Autodesk Fusion 360 part; units mm, degrees
sketch "Sketch1" plane through (0, 0, 0) normal (0, 1, 0) x (1, 0, 0)
  line L0 (0, 0) -> (70, 0)
  line L1 (70, 0) -> (70, -50)
  line L2 (70, -50) -> (0, -50)
  line L3 (0, -50) -> (0, 0)
  circle A0 centre (0, -50) radius 2
  circle A1 centre (0, 0) radius 2
  circle A2 centre (70, 0) radius 2
  circle A3 centre (70, -50) radius 2
  line L4 (0, 4) -> (70, 4)
  line L5 (74, 0) -> (74, -50)
  line L6 (70, -54) -> (0, -54)
  line L7 (-4, -50) -> (-4, 0)
  arc A4 (-4, -50) -> (0, -54) centre (0, -50) ccw
  arc A5 (0, 4) -> (-4, 0) centre (0, 0) ccw
  arc A6 (70, -54) -> (74, -50) centre (70, -50) ccw
  arc A7 (74, 0) -> (70, 4) centre (70, 0) ccw
  dimension "d1" = 70
  dimension "d2" = 50
  dimension "d3" = 4
  dimension "d4" = 4
  dimension "d5" = 4
  dimension "d6" = 4
  dimension "d8" = 4
  dimension "d9" = 4
  dimension "d10" = 4
  dimension "d11" = 4
extrude "Extrude1" add sketch "Sketch1" along normal blind 1 contours L0 L1 L2 L3 A0 A1 A2 A3 | L4 L5 L6 L7 A4 A5 A6 A7
sketch "Sketch2" plane through (0, 0, 0) normal (0, -1, 0) x (1, 0, 0)
  circle A0 centre (0, 0) radius 2
  circle A1 centre (0, 50) radius 2
  circle A2 centre (70, 0) radius 2
  circle A3 centre (70, 50) radius 2
  arc A4 (74, 50) -> (70, 54) centre (70, 50) ccw
  line L0 (70, 54) -> (0, 54)
  arc A5 (0, 54) -> (-4, 50) centre (0, 50) ccw
  line L1 (-4, 50) -> (-4, 0)
  arc A6 (-4, 0) -> (0, -4) centre (0, 0) ccw
  line L2 (0, -4) -> (70, -4)
  arc A7 (70, -4) -> (74, 0) centre (70, 0) ccw
  line L3 (74, 0) -> (74, 50)
  line L4 (10, 54) -> (10, -4)
  line L5 (56.228, 54) -> (56.228, -4)
  circle A8 centre (10, 32.046) radius 1.15
  circle A9 centre (56.228, 38.142) radius 1.15
  circle A10 centre (56.228, 25.188) radius 1.15
  line L6 (10, 45) -> (56.228, 45)
  line L7 (56.228, 45) -> (56.228, 5)
  line L8 (56.228, 5) -> (10, 5)
  line L9 (10, 5) -> (10, 45)
  line L10 (10, 25) -> (-4, 25)
  circle A11 centre (10, 32.046) radius 3.15
  circle A12 centre (56.228, 38.142) radius 3.15
  circle A13 centre (56.228, 25.188) radius 3.15
  line L11 (56.228, 38.142) -> (56.228, 25.188)
  circle A14 centre (53.728, 31.665) radius 1.5
  circle A15 centre (58.728, 31.665) radius 1.5
  line L12 (0, 50) -> (70, 50)
  line L13 (32.5, 51.5) -> (37.5, 51.5)
  line L14 (37.5, 51.5) -> (37.5, 48.5)
  line L15 (37.5, 48.5) -> (32.5, 48.5)
  line L16 (32.5, 48.5) -> (32.5, 51.5)
  line L17 (32.5, 51.5) -> (37.5, 48.5)
  line L18 (32.5, 48.5) -> (37.5, 51.5)
  line L19 (53.728, 31.665) -> (58.728, 31.665)
  point P0 (35, 50)
  point P1 (35, 50)
  point P2 (56.228, 31.665)
  point P3 (56.228, 31.665)
  dimension "d15" = 10
  dimension "d16" = 46.228
  dimension "d18" = 6.096
  dimension "d19" = 12.954
  dimension "d20" = 6.858
  dimension "d21" = 2.3
  dimension "d22" = 2.3
  dimension "d23" = 2.3
  dimension "d24" = 40
  dimension "d25" = 90
  dimension "d26" = 2
  dimension "d27" = 2
  dimension "d28" = 2
  dimension "d32" = 3
  dimension "d33" = 3
  dimension "d34" = 5
  dimension "d40" = 3
  dimension "d41" = 5
extrude "Extrude2" add sketch "Sketch2" along normal blind 5 contours L4 A8 L9 A11 | L4 A8 L9 A11 | L5 A9 L7 A12 L11 | L5 A9 L7 A12 L11 | L5 A10 L7 A13 L11 | L5 A10 L7 A13 L11
extrude "Extrude3" cut sketch "Sketch2" against normal blind 5 contours A14 | L12 L16 L17 | L12 L16 L18 | A15 | L12 L14 L18 | L12 L14 L17 | L15 L17 L18 | L13 L17 L18
Build history of the part. All positions in model axes, mm. A direction names the side the tool comes from. Give positions to 0.01 mm unless a question says otherwise; leave off trailing zeros. Loops run counter-clockwise (first coordinate to the right, second up) from the corner with the lowest first, then second, coordinate; pieces in that order, holes last. Notation, with made-up numbers: (28.25, -21.75) -> (59.25, -21.75) arc R22 cw to (59.25, 9.25) -> close; hole circle Ø11 at (-33, 85). An arc over 180 degrees is marked (long way). Answer in a Markdown table with one row per item.
Item 1: Slice it at A-A on y = -1.4. Write the cut outline in (x, z), plus the area to 3 significant figures.
Findings below:
| item | result |
|---|---|
| outline | circle Ø6.3 at (10, 32.05); circle Ø6.3 at (56.23, 25.19); circle Ø6.3 at (56.23, 38.14); hole circle Ø2.3 at (10, 32.05); hole circle Ø2.3 at (56.23, 25.19); hole circle Ø2.3 at (56.23, 38.14) |
| area | 81.1 mm² |
Item 2: Mould opens along X. For faces 1 (the cylindrical face through (71.908, 0.493, 0.601)), 2 (the cylindrical face through (-2.859, 0.493, -2.797)), 3 (the flat face through (34, 1, 25)) say: pulls with the +X half, pulls with the -X half, needs draft (parallel to the pull), parting line crosses it, or undercut.
Findings below:
| item | result |
|---|---|
| face 1 | undercut |
| face 2 | pulls with the -X half |
| face 3 | needs draft |
Item 3: Tool access for faces 4 (the cylindrical face through (60.159, 0.493, 32.116)), 5 (the flat face through (56, 0, 38)): list every direction of +Z, -Z, +X, -X, +Y, -Y with a clear straight run to the whole face (end or side of a thin tool).
Findings below:
| item | result |
|---|---|
| face 4 | +Y, -Y |
| face 5 | -Y |
Item 4: Flat gauge pins, fed straight in: P1, Ø4.5, axis at x = 0, z = 0, coming from the -Y side; P2, Ø1.8, axis at x = 53.728, z = 31.665, coming from the +Y side; P3, Ø3, axis at y = -4.5, z = 23, coming from the -X side. Where does each tip first touch, or does it go through?
Findings below:
| item | result |
|---|---|
| P1 | stops at y = 0 |
| P2 | passes through |
| P3 | stops at x = 53.15 |
Item 5: Probe line 1 along Z through (x, y) = (0, 0.3); line 2 along X through (y, z) = (0.65, 50); line 3 along X through (y, z) = (0.75, 0). List the from-to ranges inside material, lowest first. Write a range as [from, to].
Findings below:
| item | result |
|---|---|
| line 1 | z = [-4, -2], [2, 48], [52, 54] |
| line 2 | x = [-4, -2], [2, 32.5], [37.5, 68], [72, 74] |
| line 3 | x = [-4, -2], [2, 68], [72, 74] |
Item 6: Slice it at C-C on x = 10. Write the cut outline in (y, z).
Findings below:
| item | result |
|---|---|
| outline | (-5, 28.9) -> (0, 28.9) -> (0, -4) -> (1, -4) -> (1, 54) -> (0, 54) -> (0, 35.2) -> (-5, 35.2) -> (-5, 33.2) -> (0, 33.2) -> (0, 30.9) -> (-5, 30.9) -> close |
Item 7: Slice it at B-B on x = 1. Write the cut outline in (y, z), plus the area to 3 significant figures.
Findings below:
| item | result |
|---|---|
| outline | (0, -4) -> (1, -4) -> (1, -1.73) -> (0, -1.73) -> close; (0, 1.73) -> (1, 1.73) -> (1, 48.27) -> (0, 48.27) -> close; (0, 51.73) -> (1, 51.73) -> (1, 54) -> (0, 54) -> close |
| area | 51.1 mm² |
